For this review, use the dimensioned drawing (mm, ordinates from the lowest corner) and the shaded views. A direction names the side the tool comes from. Coordinates: 2 decimals unless noted, no trailing zeros. Loops run counter-clockwise (first coordinate to the right, second up) from the corner with the lowest first, then second, coordinate; pieces in that order, holes last. Notation, with made-up numbers: (-19.75, 61.25) - (35.25, 61.25) arc R28 ccw to (35.25, 86.25) - close; hole circle Ø10 at (-40, 33). An arc over 180 degrees is marked (long way). One line per item, written item: value. Start each with the question number.
1. Insertion check: P1, Ø2, axis at x = 11.5, z = 9, coming from the -Y side; P2, Ø10.5, axis at x = 34, y = 22.5, coming from the -Z side. Each pin has a flat end and moves straight along its axis. Give the tip position at first contact, or say it passes through.
2. We need section A-A, the plane z = 8.5. Give the boundary of the cut face in (x, y).
3. For the marked faces 1 and 2, list the 3-axis set-ups (+Z, -Z, +X, -X, +Y, -Y) from which the entire face can be reached by the end or side of a thin tool; tool diameter is ignored.
4. We need section B-B, the plane y = 65. Give the boundary of the cut face in (x, z), then the cut area to 3 significant figures.
5. We need section C-C, the plane x = 24. Give the boundary of the cut face in (y, z).
6. To check wall thickness, follow line 1 (X direction, y = 8.5, z = 6); line 2 (Z direction, x = 41.5, y = 36.5). State the ranges of each line that lie inside material, in increasing order.
7. Mouldability with a two-part tool opening along X and no side actions: class the marked faces 3, 4, 5 and 6 as +X half, -X half, draft (parallel to the pull), parting line (faces both ways), or undercut.
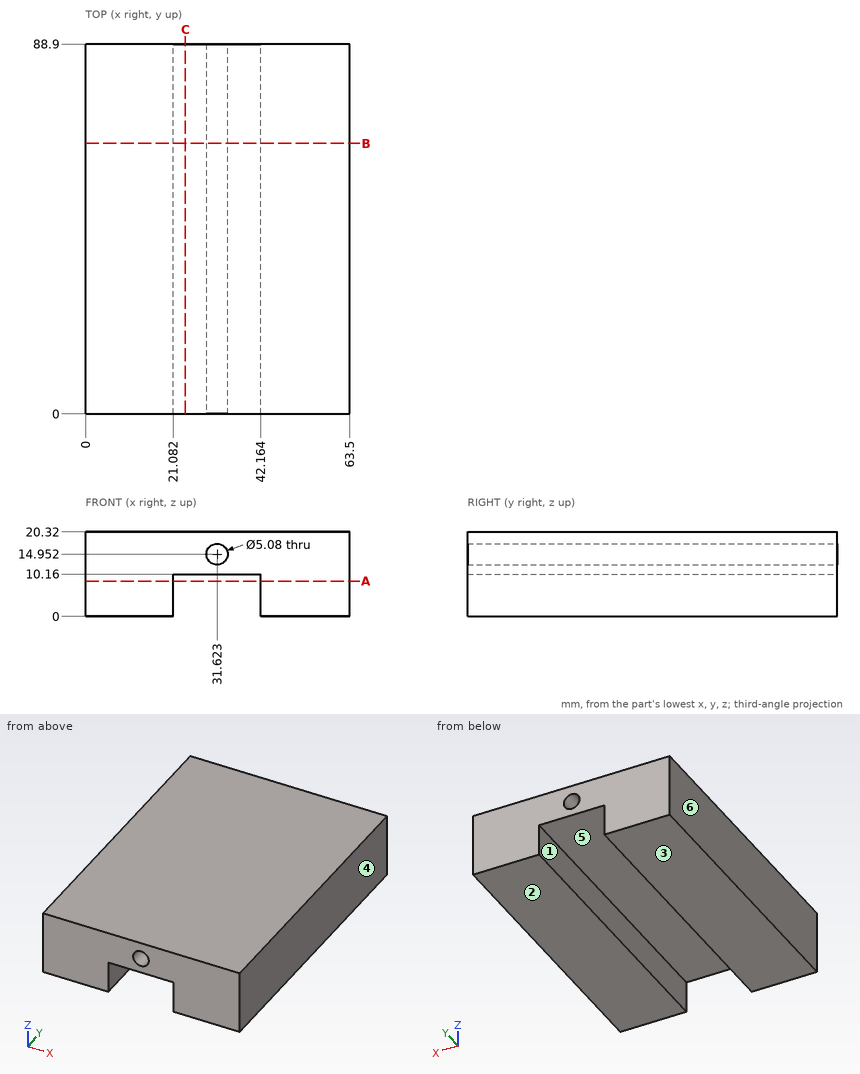
Findings below:
1. P1: y = 0
1. P2: z = 10.16
2. outline: (0, 0) - (21.08, 0) - (21.08, 88.9) - (0, 88.9) - close; (42.16, 0) - (63.5, 0) - (63.5, 88.9) - (42.16, 88.9) - close
3. face 1: -Z, +Y, -Y
3. face 2: -Z, +X, -X, +Y, -Y
4. outline: (0, 0) - (21.08, 0) - (21.08, 10.16) - (42.16, 10.16) - (42.16, 0) - (63.5, 0) - (63.5, 20.32) - (0, 20.32) - close; hole circle Ø5.08 at (31.62, 14.95)
4. area: 1,060 mm2
5. outline: (0, 10.16) - (88.9, 10.16) - (88.9, 20.32) - (0, 20.32) - close
6. line 1: 0 to 21.08, 42.16 to 63.5
6. line 2: 10.16 to 20.32
7. face 3: draft
7. face 4: +X half
7. face 5: undercut
7. face 6: -X half
